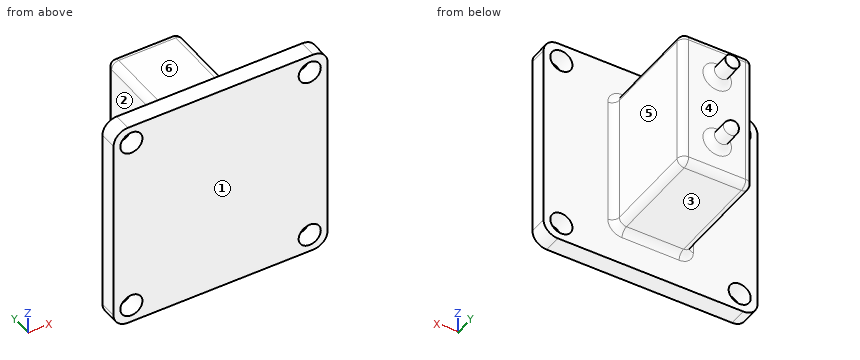
from build123d import *

# Parameters (mm, degrees)
SKETCH1_W           = 60
SKETCH1_H           = 60
SKETCH1_R           = 3.1
BOSS_EXTRUDE1_DEPTH = 5
SKETCH4_W           = 20
SKETCH4_H           = 40
BOSS_EXTRUDE3_DEPTH = 30
SKETCH2_R           = 2
BOSS_EXTRUDE2_DEPTH = 8
FILLET1_R           = 2
FILLET2_R           = 4
FILLET3_R           = 2


with BuildPart() as part:
    # Sketch1 → Boss-Extrude1 (new body)
    with BuildSketch(Plane(origin=(0, 0, 0), x_dir=(1, 0, 0), z_dir=(0, 1, 0))):
        Rectangle(SKETCH1_W, SKETCH1_H)
        with Locations((-25, 25)):
            Circle(SKETCH1_R, mode=Mode.SUBTRACT)
        with Locations((-25, -25)):
            Circle(SKETCH1_R, mode=Mode.SUBTRACT)
        with Locations((25, -25)):
            Circle(SKETCH1_R, mode=Mode.SUBTRACT)
        with Locations((25, 25)):
            Circle(SKETCH1_R, mode=Mode.SUBTRACT)
    extrude(amount=BOSS_EXTRUDE1_DEPTH)

    # Sketch4 → Boss-Extrude3 (add)
    with BuildSketch(Plane(origin=(0, 5, 0), x_dir=(1, 0, 0), z_dir=(0, 1, 0))):
        Rectangle(SKETCH4_W, SKETCH4_H)
    extrude(amount=BOSS_EXTRUDE3_DEPTH)

    # Sketch2 → Boss-Extrude2 (add)
    with BuildSketch(Plane(origin=(0, 35, 0), x_dir=(1, 0, 0), z_dir=(0, 1, 0))):
        with Locations((0, 10)):
            Circle(SKETCH2_R)
        with Locations((0, -10)):
            Circle(SKETCH2_R)
    extrude(amount=BOSS_EXTRUDE2_DEPTH)

    # Fillet1
    fillet1_edges = [part.edges().sort_by_distance(p)[0] for p in [
        (-2, 35, 10),
        (-2, 35, -10),
        (-2, 43, -10),
    ]]
    fillet(fillet1_edges, radius=FILLET1_R)

    # Fillet2
    fillet2_edges = [part.edges().sort_by_distance(p)[0] for p in [
        (30, 2.5, 30),
        (-30, 2.5, 30),
        (-30, 2.5, -30),
        (30, 2.5, -30),
    ]]
    fillet(fillet2_edges, radius=FILLET2_R)

    # Sketch3 → Cut-Revolve3 (revolve, cut)
    with BuildSketch(Plane(origin=(0, 0, 0), x_dir=(0, 0, -1), z_dir=(1, 0, 0))):
        Polygon((-10, 43), (-10, 44), (-12, 44), (-12, 41.845299462), align=None)
    revolve(axis=Axis((0, 43, 10), (0, 1, 0)), mode=Mode.SUBTRACT)

    # Fillet3
    fillet3_edges = [part.edges().sort_by_distance(p)[0] for p in [
        (10, 5, 0),
        (10, 20, 20),
        (0, 5, -20),
        (10, 20, -20),
        (-10, 5, 0),
        (-10, 20, -20),
        (0, 5, 20),
        (-10, 20, 20),
        (10, 35, 0),
        (0, 35, -20),
        (-10, 35, 0),
        (0, 35, 20),
    ]]
    fillet(fillet3_edges, radius=FILLET3_R)


solid = part.part
Design review of the part built by this model. Coordinates are the model's own, in mm. Face numbers are marked on the shaded views. A direction names the side the tool comes from. Round coordinates to 2 decimals unless told otherwise and drop trailing zeros. Write each loop counter-clockwise with the first axis right and the second up, starting at its lowest first coordinate (ties: lowest second). Pieces come first, ordered by that corner, then holes. Notation, with made-up numbers: (-11.75, 88) - (-4.75, 88) arc R27 ccw to (-4.75, 117) - close; hole circle Ø10 at (85, -28.5). An arc over 180 degrees is marked (long way). Use a Markdown table: item, result. Add a question column.
1. Mouldability with a two-part tool opening along Z and no side actions: class the marked faces 3, 4, 5 and 6 as +Z half, -Z half, draft (parallel to the pull), parting line (faces both ways), or undercut.
2. Wall thickness on probe 1 along Z at (x, y) = (25, 1); probe 2 along Y at (x, z) = (-17.5, 17.5): over which ranges is each line inside the solid? List them lowest first.
3. For the marked faces 1 and 2, list the 3-axis set-ups (+Z, -Z, +X, -X, +Y, -Y) from which the entire face can be reached by the end or side of a thin tool; tool diameter is ignored.
4. Clearance check with flat-ended pins moving along their axes: pin 1 (3 mm diameter, centred on x = 7.5, z = -4.5, fed in from +Y); pin 2 (12 mm diameter, centred on x = -7, y = 25, fed in from +Z); pin 3 (1 mm diameter, centred on x = -3, y = 6, fed in from -Z). State where each tip first meets the part, or that it passes through.
5. We need section A-A (x = 25). State the section outline as (y, z) points, then the cut area to 3 significant figures.
6. We need section C-C (z = -25). State the section outline as (x, y) points.
7. We need section B-B (y = 4). State the section outline as (x, z) points, then the cut area to 3 significant figures.
8. We need section D-D (z = -5). State the section outline as (x, y) points.
Output:
| question | item | result |
|---|---|---|
| 1 | face 3 | -Z half |
| 1 | face 4 | undercut |
| 1 | face 5 | draft |
| 1 | face 6 | +Z half |
| 2 | probe 1 | z = -30 to -28.1, -21.9 to 21.9, 28.1 to 30 |
| 2 | probe 2 | y = 0 to 5 |
| 3 | face 1 | +Z, -Z, +X, -X, -Y |
| 3 | face 2 | +Z, -Z, -X, +Y |
| 4 | pin 1 | stops at y = 35 |
| 4 | pin 2 | stops at z = 20 |
| 4 | pin 3 | stops at z = -20.68 |
| 5 | outline | (0, -30) - (5, -30) - (5, -28.1) - (0, -28.1) - close; (0, -21.9) - (5, -21.9) - (5, 21.9) - (0, 21.9) - close; (0, 28.1) - (5, 28.1) - (5, 30) - (0, 30) - close |
| 5 | area | 238 mm2 |
| 6 | outline | (-30, 0) - (-28.1, 0) - (-28.1, 5) - (-30, 5) - close; (-21.9, 0) - (21.9, 0) - (21.9, 5) - (-21.9, 5) - close; (28.1, 0) - (30, 0) - (30, 5) - (28.1, 5) - close |
| 7 | outline | (-30, -26) arc R4 ccw to (-26, -30) - (26, -30) arc R4 ccw to (30, -26) - (30, 26) arc R4 ccw to (26, 30) - (-26, 30) arc R4 ccw to (-30, 26) - close; hole circle Ø6.2 at (-25, -25); hole circle Ø6.2 at (-25, 25); hole circle Ø6.2 at (25, -25); hole circle Ø6.2 at (25, 25) |
| 7 | area | 3,470 mm2 |
| 8 | outline | (-30, 0) - (30, 0) - (30, 5) - (12, 5) arc R2 cw to (10, 7) - (10, 33) arc R2 ccw to (8, 35) - (-8, 35) arc R2 ccw to (-10, 33) - (-10, 7) arc R2 cw to (-12, 5) - (-30, 5) - close |
